```python
from build123d import *

# Parameters (mm, degrees)
SKETCH1_W          = 50.8
SKETCH1_H          = 258.7625
SKETCH1_R          = 12.7
EXTRUDE1_DEPTH     = 12.7
CUT_EXTRUDE1_DEPTH = 135.275194476


with BuildPart() as part:
    # Sketch1 → Extrude1 (new, symmetric)
    with BuildSketch(Plane.XY):
        Rectangle(SKETCH1_W, SKETCH1_H)
        with Locations((0, 103.98125)):
            Circle(SKETCH1_R, mode=Mode.SUBTRACT)
        with Locations((0, -103.98125)):
            Circle(SKETCH1_R, mode=Mode.SUBTRACT)
    extrude(amount=EXTRUDE1_DEPTH, both=True)

    # Sketch2 → Cut-Extrude1 (cut, through all)
    with BuildSketch(Plane.XY.offset(12.7)):
        Polygon((-6.35, 129.38125), (-25.4, 110.33125), (-25.4, 129.38125), align=None)
        Polygon((6.35, 129.38125), (25.4, 110.33125), (25.4, 129.38125), align=None)
        Polygon((-25.4, -110.33125), (-6.35, -129.38125), (-25.4, -129.38125), align=None)
        Polygon((25.4, -110.33125), (25.4, -129.38125), (6.35, -129.38125), align=None)
    extrude(amount=-CUT_EXTRUDE1_DEPTH, mode=Mode.SUBTRACT)


solid = part.part
```
Build history of the part. All positions in model axes, mm. Coordinates: 2 decimals unless noted, no trailing zeros. Order: outer loops, then holes, each group sorted by start corner. A loop starts at its lowest first (then second) coordinate and runs counter-clockwise, first axis right, second up.
Item 1: Saw through at C-C on x = 10. List the corners of the cut face in (y, z).
Filled in:
outline: (-125.73, -12.7) - (-111.81, -12.7) - (-111.81, 12.7) - (-125.73, 12.7) - close; (-96.15, -12.7) - (96.15, -12.7) - (96.15, 12.7) - (-96.15, 12.7) - close; (111.81, -12.7) - (125.73, -12.7) - (125.73, 12.7) - (111.81, 12.7) - close
Item 2: Drop a flat-ended pin along its axis: pin 1 Ø1.5 at (x, z) = (16.5, -6.5) entering from +Y. Give the stop position or say it passes through.
Filled in:
pin 1: stops at y = 119.98
Item 3: Saw through at B-B on z = 10. List the corners of the cut face in (x, y), then the cut area to 3 significant figures.
Filled in:
outline: (-25.4, -110.33) - (-6.35, -129.38) - (6.35, -129.38) - (25.4, -110.33) - (25.4, 110.33) - (6.35, 129.38) - (-6.35, 129.38) - (-25.4, 110.33) - close; hole circle Ø25.4 at (0, -103.98); hole circle Ø25.4 at (0, 103.98)
area: 11,400 mm2
Item 4: Drill centre lines: L1, parallel to Y at x = 0, z = -2; L2, parallel to Y at x = 1.5, z = 2.5; L3, parallel to X at y = -100, z = 2.75. Where is each one in solid material? Low to high.
Filled in:
L1: y = -129.38 to -116.68, -91.28 to 91.28, 116.68 to 129.38
L2: y = -129.38 to -116.59, -91.37 to 91.37, 116.59 to 129.38
L3: x = -25.4 to -12.06, 12.06 to 25.4
Item 5: Mould opens along Y. For faces 1 (the flat face through (-15.74, 119.99, 0.18)), 2 (the flat face through (0, 2, 12.7)), 3 (the cylindrical face through (-2.753, 91.583, -0.178)) say: released by +Y, released by -Y, zero draft, split by the parting line, or undercut.
Filled in:
face 1: released by +Y
face 2: zero draft
face 3: undercut
Item 6: Saw through at A-A on x = 0. List the corners of the cut face in (y, z).
Filled in:
outline: (-129.38, -12.7) - (-116.68, -12.7) - (-116.68, 12.7) - (-129.38, 12.7) - close; (-91.28, -12.7) - (91.28, -12.7) - (91.28, 12.7) - (-91.28, 12.7) - close; (116.68, -12.7) - (129.38, -12.7) - (129.38, 12.7) - (116.68, 12.7) - close
